Autodesk Inventor part; units mm, degrees
ref_plane "YZ Plane" through (0, 0, 0) normal (1, 0, 0) x (0, 1, 0)
ref_plane "XY Plane" through (0, 0, 0) normal (0, 0, 1) x (1, 0, 0)
sketch "Эскиз1" plane through (0, 0, 0) normal (0, 1, 0) x (-1, 0, 0)
  circle A0 centre (-0.8899, -31.6552) radius 10
  circle A1 centre (-0.8899, -31.6552) radius 20
  line L0 (-0.8899, -11.6552) -> (-0.8899, 108.3448)
  line L1 (-0.8899, -31.6552) -> (78.1589, -77.294)
  line L2 (-0.8899, -31.6552) -> (90.3878, -31.6552) construction
  line L3 (78.1589, -77.294) -> (120.2106, -101.5726)
  line L4 (-0.8899, -31.6552) -> (116.9091, -31.6552) construction
  line L5 (-0.8899, -31.6552) -> (-104.8129, -91.6552)
  line L6 (-0.8899, -31.6552) -> (119.1101, -31.6552) construction
  line L7 (-104.8129, -91.6552) -> (-122.5612, -101.9021)
  line L8 (-122.5612, -101.9021) -> (-117.5612, -110.5624)
  line L9 (-117.5612, -110.5624) -> (4.1101, -40.3154)
  line L10 (-122.5612, -101.9021) -> (-127.5612, -93.2419)
  line L11 (-127.5612, -93.2419) -> (-5.8899, -22.9949)
  line L12 (120.2106, -101.5726) -> (125.2106, -92.9123)
  line L13 (125.2106, -92.9123) -> (4.1101, -22.9949)
  line L14 (120.2106, -101.5726) -> (7.7704, -36.6552)
  line L15 (-0.8899, 108.3448) -> (-10.8899, 108.3448)
  line L16 (-10.8899, 108.3448) -> (9.1101, 108.3448)
  line L17 (9.1101, 108.3448) -> (9.1101, -31.6552)
  line L18 (-10.8899, 108.3448) -> (-10.8899, -31.6552)
  line L19 (120.2106, -101.5726) -> (115.2106, -110.2328)
  line L20 (115.2106, -110.2328) -> (-5.8899, -40.3154)
  line L21 (9.1101, 108.3448) -> (9.1101, 88.3448)
  line L22 (9.1101, 88.3448) -> (-10.8899, 88.3448)
  line L23 (-10.8899, 108.3448) -> (9.1101, 88.3448)
  line L24 (9.1101, 108.3448) -> (-10.8899, 88.3448)
  line L25 (-0.8899, 98.3448) -> (-0.8899, 93.3448)
  line L26 (-0.8899, 93.3448) -> (4.1101, 93.3448)
  line L27 (4.1101, 103.3448) -> (-5.8899, 103.3448)
  line L28 (-5.8899, 103.3448) -> (-5.8899, 93.3448)
  line L29 (-5.8899, 93.3448) -> (-0.8899, 93.3448)
  line L30 (-127.5612, -93.2419) -> (-110.2407, -83.2419)
  line L31 (-110.2407, -83.2419) -> (-100.2407, -100.5624)
  line L32 (-127.5612, -93.2419) -> (-100.2407, -100.5624)
  line L33 (-117.5612, -110.5624) -> (-110.2407, -83.2419)
  line L34 (-113.9009, -96.9021) -> (-118.2311, -99.4021)
  line L35 (-118.2311, -99.4021) -> (-115.7311, -103.7322)
  line L36 (-115.7311, -103.7322) -> (-107.0708, -98.7322)
  line L37 (-107.0708, -98.7322) -> (-112.0708, -90.072)
  line L38 (-112.0708, -90.072) -> (-120.7311, -95.072)
  line L39 (-120.7311, -95.072) -> (-118.2311, -99.4021)
  circle A2 centre (-113.9009, -96.9021) radius 2
  line L40 (120.2106, -101.5726) -> (111.5503, -96.5726)
  line L41 (111.5503, -96.5726) -> (102.8901, -91.5726)
  line L42 (102.8901, -91.5726) -> (107.2202, -94.0726)
  line L43 (107.2202, -94.0726) -> (104.7202, -98.4027)
  line L44 (104.7202, -98.4027) -> (113.3805, -103.4027)
  line L45 (113.3805, -103.4027) -> (118.3805, -94.7424)
  line L46 (118.3805, -94.7424) -> (109.7202, -89.7424)
  line L47 (109.7202, -89.7424) -> (107.2202, -94.0726)
  line L48 (104.7202, -98.4027) -> (118.3805, -94.7424)
  circle A3 centre (111.5503, -96.5726) radius 2
  circle A4 centre (-118.2311, -99.4021) radius 2
  line L49 (-113.9009, -96.9021) -> (-116.2311, -92.4739)
  line L50 (-116.2311, -92.4739) -> (-125.0612, -97.572)
  line L51 (-113.9009, -96.9021) -> (-111.4009, -101.2322)
  line L52 (-111.4009, -101.2322) -> (-120.0612, -106.2322)
  line L53 (-125.0612, -97.572) -> (-120.0612, -106.2322)
  line L54 (-5.8899, 103.3448) -> (-5.8899, 108.3448)
  line L55 (4.1101, 103.3448) -> (4.1101, 108.3448)
  line L56 (4.1101, 103.3448) -> (4.1101, 98.3448)
  line L57 (4.1101, 98.3448) -> (-5.8899, 98.3448)
  circle A5 centre (-0.8899, 103.3448) radius 2
  line L58 (118.3805, -94.7424) -> (122.7106, -97.2424)
  line L59 (113.3805, -103.4027) -> (117.7106, -105.9027)
  line L60 (111.5503, -96.5726) -> (109.0503, -100.9027)
  line L61 (111.5503, -96.5726) -> (114.0503, -92.2424)
  circle A6 centre (115.8805, -99.0726) radius 2
  point P0 (0, 0)
  point P1 (-0.8899, 101.3448)
  point P2 (1.1101, 103.3448)
  point P3 (-0.8899, 103.3448)
  dimension "d0" = 20
  dimension "d1" = 40
  dimension "d2" = 120
  dimension "d3" = 30
  dimension "d4" = 120
  dimension "d5" = 150
  dimension "d6" = 10
  dimension "d7" = 10
  dimension "d8" = 10
  dimension "d9" = 10
  dimension "d13" = 20
  dimension "d38" = 5
  dimension "d39" = 20
  dimension "d40" = 5
  dimension "d41" = 4
  dimension "d42" = 10
  dimension "d43" = 10
  dimension "d44" = 5
  dimension "d45" = 10
  dimension "d46" = 10
  dimension "d47" = 10
  dimension "d48" = 4
  dimension "d53" = 4
  dimension "d58" = 4
  dimension "d63" = 4
ref_plane "РабПлоскость1" through (0, 15, 0) normal (0, 1, 0) x (-1, 0, 0)
sketch "Эскиз2" plane through (0, 15, 0) normal (0, 1, 0) x (-1, 0, 0)
  circle A0 centre (-0.8908, -31.6557) radius 10
  circle A1 centre (-0.8908, -31.6557) radius 20
  circle A2 centre (-0.8908, -31.6557) radius 11
  point P0 (0, 0)
  dimension "d11" = 20
  dimension "d12" = 40
  dimension "d68" = 22
extrude "Выдавливание1" add sketch "Эскиз2" against normal blind 6 contours A1 | A2
ref_plane "РабПлоскость2" through (0.8899, 0, -31.6552) normal (0.5, 0, 0.866) x (0.866, 0, -0.5)
ref_plane "РабПлоскость3" through (-120.2106, 0, -101.5726) normal (0.5, 0, -0.866) x (0.866, 0, 0.5)
sketch "Эскиз4" plane through (0.8899, 0, -31.6552) normal (0.5, 0, 0.866) x (0.866, 0, -0.5)
  line L0 (20.0011, 15) -> (-19.9989, 15)
  line L1 (-19.9989, 9) -> (20.0011, 9)
  line L2 (20.0011, 15) -> (20.0011, 9)
  line L3 (20.0011, 15) -> (140.5253, 0)
  line L4 (140.5253, 0) -> (120.5253, 0)
  line L5 (120.5253, 0) -> (20.0011, 9)
  line L6 (20.0011, 15) -> (19.0011, 15)
  line L7 (20.0011, 15) -> (18.0011, 15)
  line L8 (18.0011, 15) -> (18.0011, 9)
  line L9 (20.0011, 9) -> (18.0011, 9)
  point P0 (-16.5982, 0)
  point P1 (-17.3194, 15)
  point P2 (-17.3194, 15)
  dimension "d22" = 20
  dimension "d25" = 2
extrude "Выдавливание3" add sketch "Эскиз4" along normal mid plane 15
ref_plane "РабПлоскость4" through (0.8899, 0, -11.6552) normal (1, 0, 0) x (0, 0, 1)
sketch "Эскиз5" plane through (0.8899, 0, -11.6552) normal (1, 0, 0) x (0, 0, 1)
  point P0 (11.6552, 0)
sketch "Эскиз6" plane through (0.8899, 0, -11.6552) normal (1, 0, 0) x (0, 0, 1)
  line L0 (-40.0005, -15) -> (-0.0005, -15)
  line L1 (-0.0005, -15) -> (119.9781, 0)
  line L2 (119.9781, 0) -> (99.9781, 0)
  line L3 (-0.0005, -9) -> (-40.0005, -9)
  line L4 (99.9781, 0) -> (-0.0005, -9)
  line L5 (-0.0005, -9) -> (-2.0005, -9)
  line L6 (-2.0005, -9) -> (-2.0005, -15)
  line L7 (-0.0005, -15) -> (-2.0005, -15)
  point P0 (11.6552, 0)
  point P1 (-35.766, -15)
  point P2 (-22.7756, -15)
  point P3 (-22.7756, -9)
  point P4 (-35.766, -9)
  dimension "d29" = 20
  dimension "d30" = 2
extrude "Выдавливание4" add sketch "Эскиз6" along normal mid plane 15
sketch "Эскиз7" plane through (-120.2106, 0, -101.5726) normal (0.5, 0, -0.866) x (0.866, 0, 0.5)
  line L0 (119.8354, -15) -> (142.6104, -15)
  line L1 (119.8354, -15) -> (0, 0)
  line L2 (0, 0) -> (20, 0)
  line L3 (142.6104, -9) -> (119.8354, -9)
  line L4 (20, 0) -> (119.8354, -9)
  line L5 (119.8354, -9) -> (121.8354, -9)
  line L6 (121.8354, -9) -> (121.8354, -15)
  line L7 (119.8354, -15) -> (121.8354, -15)
  point P0 (154.8917, 0)
  point P1 (142.6094, -15)
  point P2 (142.6094, -9)
  dimension "d33" = 20
  dimension "d34" = 2
extrude "Выдавливание5" add sketch "Эскиз7" along normal mid plane 15
extrude "Выдавливание8" add sketch "Эскиз1" along normal blind 3 contours L50 L39 A4 L7 L10 | L38 L49 A2 L32 | L32 A2 L7 A4 L39 | L8 L7 A4 L35 L52 | L35 A4 L7 A2 L33 | L33 A2 L51 L36 | A2 L49 L32 | L32 L7 A2 | L33 A2 L7 | L51 A2 L33 picked at (-115.1931, -97.2034) picked at (-114.6016, -98.0289)
extrude "Выдавливание9" cut sketch "Эскиз1" along normal blind 4 contours A4 L7 L39 | L39 L7 A4 | A4 L7 L35 | L35 L7 A4
extrude "Выдавливание10" add sketch "Эскиз1" along normal blind 3 contours L55 L27 A5 L0 L16 | L56 L57 L24 | L24 L0 A5 L27 | L23 L27 A5 L0 | L57 L28 L23 | L0 A5 L27 L54 L15 | A5 L0 L27 picked at (0.232, 102.6399)
extrude "Выдавливание11" cut sketch "Эскиз1" along normal blind 3 contours A5 L0 L27 | L27 L0 A5 | A5 L27 L0 | L0 L27 A5
extrude "Выдавливание12" add sketch "Эскиз1" along normal blind 3 contours L12 L3 A6 L45 L58 | L59 L45 A6 L3 L19 | L48 A3 L61 L46 | L45 A6 L3 A3 L48 | L44 L60 A3 L3 A6 L45 | A3 L3 L48 | L48 L61 A3 | L3 A3 L60 picked at (112.8333, -96.9164)
extrude "Выдавливание13" cut sketch "Эскиз1" along normal blind 3 contours A6 L45 L3 | L3 L45 A6 | L45 L3 A6 | A6 L3 L45
sketch "Эскиз8" plane through (0, 15, 0) normal (0, 1, 0) x (1, 0, 0)
  point P0 (0, 0)
extrude "Выдавливание14" cut sketch "Эскиз2" against normal blind 10 contours A0 | A2
properties part number "axis"
Geometry: final body of the model. Coordinates: model frame, mm. A direction names the side the tool comes from. Round coordinates to 2 decimals unless told otherwise and drop trailing zeros. Order: outer loops, then holes, each group sorted by start corner. A loop starts at its lowest first (then second) coordinate and runs counter-clockwise, first axis right, second up. Notation, with made-up numbers: (36.5, -1.5) - (71.5, -1.5) arc R21 ccw to (71.5, 11.5) - close; hole circle Ø11 at (-21.5, 83). An arc over 180 degrees is marked (long way). Write item = value, one per line. Start each with the question number.
Q1. Cut plane A-A on z = -38.5. Return the cut outline in (x, y).
Q2. Cut plane C-C on z = 29. Return the cut outline in (x, y).
Q3. Cut plane B-B on x = -45. Return the cut outline in (y, z), and give its area (3 significant figures).
Q4. Ray query, line 1 (X direction, y = 7.75, z = 12); line 2 (Z direction, x = -25, y = 12.75); line 3 (Z direction, x = -58, y = 7.25). Return the intervals inside material, ascending. Write a range as from..to.
Q5. Access query for faces 5 (the flat face through (-60.318, 4.437, -66.872)), 6 (the flat face through (-52.512, 7.465, -71.147)), 7 (the flat face through (-114.267, 3, -100.495)), 8 (the flat face through (115.67, 1.814, -103.697)). Directions: +Z, -Z, +X, -X, +Y, -Y. A direction counts if a zero-diameter tool reaches every point of the face in a straight line with its end or side. Return the directions, or none.
Q6. Pull-direction query (X, two-part tool) for faces 1 (the flat face through (0.785, 4.437, 39.033)), 2 (the flat face through (61.533, 7.535, -58.008)), 3 (the flat face through (62.297, 4.437, -67.23)), 4 (the flat face through (-8, 9, -40)); classes: +X half, -X half, draft (parallel to the pull), parting line (faces both ways), or undercut.
Q7. Pin query (flat end, axial travel): pin 1 (8 mm diameter, centred on x = -20.5, y = 8, fed in from -Z); pin 2 (5 mm diameter, centred on y = 11.5, z = -27, fed in from +X); pin 3 (11 mm diameter, centred on x = 115, z = -99, fed in from +Y). Return the tip coordinate at first contact, or that it passes through.
Outcome:
q1.outline = (-25.97, 8.4) - (-18.25, 9) - (-7.72, 9) - (-7.72, 15) - (-18.25, 15) - (-25.97, 14.16) - close; (9.5, 9) - (20.03, 9) - (27.75, 8.4) - (27.75, 14.17) - (20.03, 15) - (9.5, 15) - close
q2.outline = (-6.61, 5.34) - (8.39, 5.34) - (8.39, 9.92) - (-6.61, 9.92) - close
q3.outline = (5.64, -66.81) - (10.33, -66.81) - (11.41, -49.49) - (6.42, -49.49) - close
q3.area = 83.9 mm^2
q4.line_1 = -6.61..8.39
q4.line_2 = -55.26..-37.94
q4.line_3 = -74.32..-57
q5.face_5 = +Z, -Y
q5.face_6 = -Z, +Y, -Y
q5.face_7 = +Z, -Z, -X, +Y
q5.face_8 = -Z, +Y
q6.face_1 = draft
q6.face_2 = +X half
q6.face_3 = undercut
q6.face_4 = undercut
q7.pin_1 = -54.97
q7.pin_2 = 20.77
q7.pin_3 = 3
